Part model, mm, in its own coordinate system. A direction names the side the tool comes from. Coordinates: 2 decimals unless noted, no trailing zeros. Write each loop counter-clockwise with the first axis right and the second up, starting at its lowest first coordinate (ties: lowest second). Pieces come first, ordered by that corner, then holes. Notation, with made-up numbers: (89, -17.5) -> (132, -17.5) arc R20 cw to (132, 16.5) -> close; hole circle Ø6 at (-38.5, 22.5). An arc over 180 degrees is marked (long way). Write item = value, one per line.
from build123d import *

# Parameters (mm, degrees)
ESQUISSE1_W             = 40
ESQUISSE1_H             = 80
BOSS_EXTRU_1_DEPTH      = 1
ESQUISSE2_R             = 0.5
BOSS_EXTRU_2_DEPTH      = 80
ESQUISSE3_W             = 3
ESQUISSE3_H             = 80
ENL_V_MAT_EXTRU_1_DEPTH = 90.98333179
D_GAGEMENT_M21_D        = 2.4


with BuildPart() as part:
    # Esquisse1 → Boss.-Extru.1 (new body)
    with BuildSketch(Plane.XY):
        with Locations((20, 40)):
            Rectangle(ESQUISSE1_W, ESQUISSE1_H)
    boss_extru_1 = extrude(amount=BOSS_EXTRU_1_DEPTH)

    # Esquisse2 → Boss.-Extru.2 (add)
    with BuildSketch(Plane(origin=(0, 80, 0), x_dir=(1, 0, 0), z_dir=(0, 1, 0))):
        with BuildLine():
            Line((1, 0), (1, 1))
            ThreePointArc((1, 1), (-0.707106781, 1.707106781), (0, 0))
            Line((0, 0), (1, 0))
        make_face()
        with Locations(Location((0, 1, 0), (0, 0, 270))):
            Circle(ESQUISSE2_R, mode=Mode.SUBTRACT)
    boss_extru_2 = extrude(amount=-BOSS_EXTRU_2_DEPTH)

    # Symétrie2: Boss.-Extru.1, Boss.-Extru.2 across plane
    add(boss_extru_1.mirror(Plane.XY.offset(1)))
    add(boss_extru_2.mirror(Plane.XY.offset(1)))

    # Esquisse3 → Enlèv. mat.-Extru.1 (cut, through all)
    with BuildSketch(Plane(origin=(40, 0, 0), x_dir=(0, 0, -1), z_dir=(1, 0, 0))):
        with Locations((0.5, 40)):
            Rectangle(ESQUISSE3_W, ESQUISSE3_H)
    extrude(amount=-ENL_V_MAT_EXTRU_1_DEPTH, mode=Mode.SUBTRACT)

    # Dégagement M21 (through all)
    with Locations(Plane.XY.offset(2)):
        with Locations((30, 40)):
            Hole(D_GAGEMENT_M21_D / 2)


solid = part.part
Q1. Saw through at C-C on y = 21. Give the cut face in (x, z).
Model answer:
outline = (0, 1) -> (40, 1) -> (40, 2) -> (1, 2) -> (1, 3) arc R1 ccw (long way) to (0, 2) -> close; hole circle Ø1 at (0, 3)
Q2. Saw through at B-B on x = 30. Give the cut face in (y, z).
Model answer:
outline = (0, 1) -> (38.8, 1) -> (38.8, 2) -> (0, 2) -> close; (41.2, 1) -> (80, 1) -> (80, 2) -> (41.2, 2) -> close
Q3. Saw through at A-A on y = 40. Give the cut face in (x, z).
Model answer:
outline = (0, 1) -> (28.8, 1) -> (28.8, 2) -> (1, 2) -> (1, 3) arc R1 ccw (long way) to (0, 2) -> close; (31.2, 1) -> (40, 1) -> (40, 2) -> (31.2, 2) -> close; hole circle Ø1 at (0, 3)
Q4. Which spindle directions (+Z, -Z, +X, -X, +Y, -Y) get a long thin tool onto all of the face, cutting with end or side? Do faces 1 (the face through (19.2, 0, 1.5)), 2 (the face through (20, 41, 2)). Say none if no direction does.
Model answer:
face_1 = +Z, -Z, +X, -X, -Y
face_2 = +Z, +X, +Y, -Y
Q5. Pin check, flat tips, straight feed: pin 1 (0.5 mm diameter, centred on y = 35, z = 2.5, fed in from +X); pin 2 (0.5 mm diameter, centred on y = 54, z = 1.5, fed in from -X); pin 3 (2 mm diameter, centred on x = 30, y = 40, fed in from -Z) (3 decimals). Stop position of each tip, or through.
Model answer:
pin_1 = 1
pin_2 = 0
pin_3 = through
Q6. Probe line 1 (X direction, y = 24, z = 3); line 2 (Z direction, x = 37.5, y = 29.5); line 3 (Y direction, x = 30, z = 1.35). List the from-to ranges inside material, lowest first. Write a range as from..to.
Model answer:
line_1 = -1..-0.5, 0.5..1
line_2 = 1..2
line_3 = 0..38.8, 41.2..80
Q7. Mould opens along X. For faces 3 (the face through (19.2, 80, 1.5)), 4 (the face through (-0.683, 40.56, 3.73)), 5 (the face through (29.35, 41.01, 1.49)) say: released by +X, released by -X, zero draft, split by the parting line, or undercut.
Model answer:
face_3 = zero draft
face_4 = split by the parting line
face_5 = undercut
